Verification items for this drawing (mm, ordinates from the low corner). A direction names the side the tool comes from. Round coordinates to 2 decimals unless told otherwise and drop trailing zeros. Loops run counter-clockwise (first coordinate to the right, second up) from the corner with the lowest first, then second, coordinate; pieces in that order, holes last. Notation, with made-up numbers: (88.5, -24.75) - (104.5, -24.75) arc R14 ccw to (104.5, 1.25) - close; hole circle Ø7 at (-40, 31.25). An arc over 180 degrees is marked (long way). Use a Markdown table: item, result. Add a question column.
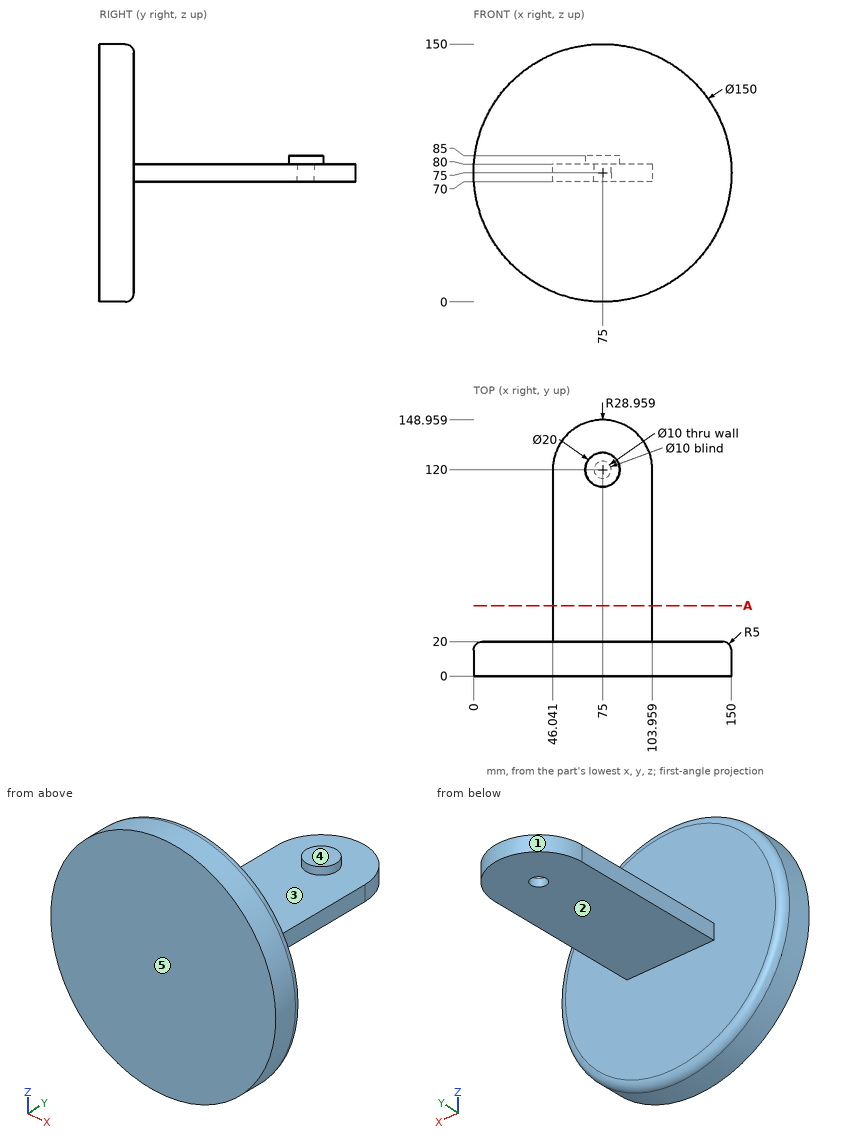
Q1. Thickness scan on line 1 along Y through (x, z) = (75, 76); line 2 along Y through (x, z) = (30.5, 38.5); line 3 along Z through (x, y) = (71, 122.5). Record the ranges inside material, lowest first.
Q2. Go/stop test with flat-tipped pins: pin 1 Ø1.5 at (x, y) = (96.5, 133.5) entering from -Z; pin 2 Ø10 at (x, y) = (70, 30) entering from +Z; pin 3 Ø5 at (x, y) = (76.5, 121.5) entering from -Z. Record where each tip stops, or that it passes through.
Q3. Set-up check for the marked faces 1 and 2: record each of +Z, -Z, +X, -X, +Y, -Y from which the full face is reachable in a straight line by a thin tool's end or side.
Q4. Release check for a two-part mould opening along Y. For the marked faces 3, 4 and 5 record: +Y half, -Y half, draft (parallel to the pull), parting line (faces both ways), or undercut.
Q5. Section check A-A on y = 41. Record the cut outline in (x, z), plus the area to 3 significant figures.
Determined:
| question | item | result |
|---|---|---|
| 1 | line 1 | y = 0 to 115, 125 to 148.96 |
| 1 | line 2 | y = 0 to 20 |
| 1 | line 3 | z = 80 to 85 |
| 2 | pin 1 | stops at z = 70 |
| 2 | pin 2 | stops at z = 80 |
| 2 | pin 3 | stops at z = 80 |
| 3 | face 1 | +Z, -Z, +Y |
| 3 | face 2 | -Z, +X, -X, +Y |
| 4 | face 3 | undercut |
| 4 | face 4 | draft |
| 4 | face 5 | -Y half |
| 5 | outline | (46.04, 70) - (103.96, 70) - (103.96, 80) - (46.04, 80) - close |
| 5 | area | 579 mm² |
